The listing builds one solid part. Answer for the finished solid, in the listing's coordinates (mm). Face numbers are marked on the shaded views. A direction names the side the tool comes from. Give positions to 0.01 mm unless a question says otherwise; leave off trailing zeros. Loops run counter-clockwise (first coordinate to the right, second up) from the corner with the lowest first, then second, coordinate; pieces in that order, holes last. Notation, with made-up numbers: (71, -25.5) - (123, -25.5) arc R30 ccw to (123, 10.5) - close; hole circle Ø2 at (51.25, 29). An arc over 180 degrees is marked (long way). Write item = value, one per line. Start each with the question number.
1) The part is cut by section D-D on z = 0. Write down the section's boundary in (x, y), plus the area to 3 significant figures.
2) The part is cut by section A-A on y = -17.75. Write down the section's boundary in (x, z).
3) Flat-ended cylindrical pins translate along their axes: P1, Ø2.5, axis at x = -38.5, y = -12, coming from the -Z side; P2, Ø10, axis at y = -21, z = 11.5, coming from the -X side; P3, Ø10, axis at x = -38.5, z = 28, coming from the -Y side; P4, Ø2.5, axis at y = -5, z = -33.5, coming from the -X side. Find the tip coordinate at first contact, or state that the pin passes through.
4) The part is cut by section B-B on z = -15.5. Write down the section's boundary in (x, y), plus the area to 3 significant figures.
5) The part is cut by section C-C on x = -40.5. Write down the section's boundary in (y, z), plus the area to 3 significant figures.
6) Consider probe 1 along X at (y, z) = (-4.25, -3.5); probe 2 along Z at (x, y) = (-40.5, -4.75); probe 3 along X at (y, z) = (-2.75, 33). Determine where each line is inside the solid, lowest interval first.
7) Which of the six approach directions +Z, -Z, +X, -X, +Y, -Y give full straight-line access (tool end or side, diameter ignored) to the marked faces 5, 6 and 7?
8) The mould has two halves that part along X. Classify the marked faces 1, 2, 3 and 4: +X half, -X half, draft (parallel to the pull), parting line (faces both ways), or undercut.
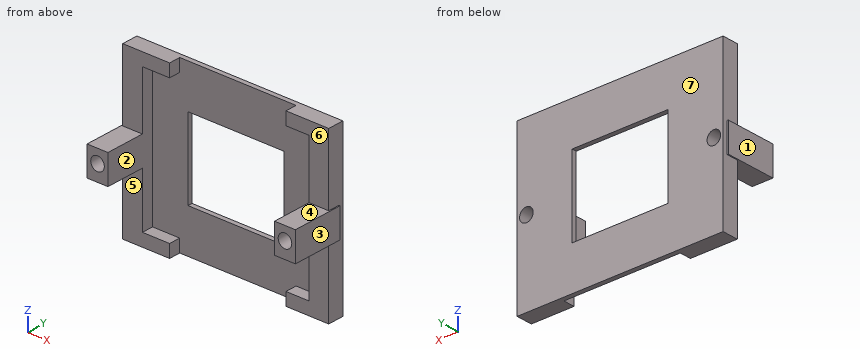
from build123d import *

# Parameters (mm, degrees)
F0_W      = 89
F0_H      = 72
F1_DEPTH  = 7
F2_W      = 72
F2_H      = 61
F3_DEPTH  = 5
F4_W      = 41.437034
F4_H      = 34.563594
F5_DEPTH  = 25
F6_W      = 50.274316
F6_H      = 5.5
F7_DEPTH  = 5
F8_W      = 9
F8_H      = 12.568578
F9_DEPTH  = 22
F10_R     = 2.9335
F11_DEPTH = 25


with BuildPart() as f1:
    # F0 (on Front) → F1 (new body)
    with BuildSketch(Plane.XZ):
        Rectangle(F0_W, F0_H)
    extrude(amount=F1_DEPTH)

    # F2 (on face) → F3 (cut)
    with BuildSketch(Plane.XZ.offset(7)):
        Rectangle(F2_W, F2_H)
    extrude(amount=-F3_DEPTH, mode=Mode.SUBTRACT)

    # F4 (on face) → F5 (cut)
    with BuildSketch(Plane.XZ.offset(2)):
        Rectangle(F4_W, F4_H)
    extrude(amount=-F5_DEPTH, mode=Mode.SUBTRACT)

    # F6 (on face) → F7 (cut)
    with BuildSketch(Plane.XZ.offset(7)):
        with Locations((0.883728, -33.25)):
            Rectangle(F6_W, F6_H)
        with Locations((0.883728, 33.25)):
            Rectangle(F6_W, F6_H)
    extrude(amount=-F7_DEPTH, mode=Mode.SUBTRACT)

    # F8 (on face) → F9 (join)
    with BuildSketch(Plane.XZ.offset(2)):
        with Locations((-40.5, -0.589152)):
            Rectangle(F8_W, F8_H)
        with Locations((40.5, -0.589152)):
            Rectangle(F8_W, F8_H)
    extrude(amount=F9_DEPTH)

    # F10 (on face) → F11 (cut)
    with BuildSketch(Plane.XZ.offset(24)):
        with Locations((-40.5, 0)):
            Circle(F10_R)
        with Locations((40.5, 0)):
            Circle(F10_R)
    extrude(amount=-F11_DEPTH, mode=Mode.SUBTRACT)


solid = f1.part
Answer below:
q1.outline = (-45, -24) - (-43.43, -24) - (-43.43, 0) - (-44.5, 0) - (-44.5, -2) - (-45, -2) - close; (-37.57, -24) - (-36, -24) - (-36, -2) - (-20.72, -2) - (-20.72, 0) - (-37.57, 0) - close; (20.72, -2) - (36, -2) - (36, -24) - (37.57, -24) - (37.57, 0) - (20.72, 0) - close; (43.43, -24) - (45, -24) - (45, -2) - (44.5, -2) - (44.5, 0) - (43.43, 0) - close
q1.area = 210 mm2
q2.outline = (-45, -6.87) - (-36, -6.87) - (-36, 5.7) - (-45, 5.7) - close; (36, -6.87) - (45, -6.87) - (45, 5.7) - (36, 5.7) - close; hole circle Ø5.87 at (-40.5, 0); hole circle Ø5.87 at (40.5, 0)
q3.P1 = -6.87
q3.P2 = through
q3.P3 = -7
q3.P4 = -44.5
q4.outline = (-44.5, -7) - (-36, -7) - (-36, -2) - (-20.72, -2) - (-20.72, 0) - (-44.5, 0) - close; (20.72, -2) - (36, -2) - (36, -7) - (44.5, -7) - (44.5, 0) - (20.72, 0) - close
q4.area = 180 mm2
q5.outline = (-24, -6.87) - (-7, -6.87) - (-7, -36) - (0, -36) - (0, -2.93) - (-24, -2.93) - close; (-24, 2.93) - (0, 2.93) - (0, 36) - (-7, 36) - (-7, 5.7) - (-24, 5.7) - close
q5.area = 577 mm2
q6.probe_1 = -45 to -36, 36 to 45
q6.probe_2 = -36 to -2.93, 2.93 to 36
q6.probe_3 = -44.5 to -24.25, 26.02 to 44.5
q7.face_5 = -Z, +X, -X, -Y
q7.face_6 = +Z, +X, -X, -Y
q7.face_7 = +Z, -Z, +X, -X, +Y
q8.face_1 = -X half
q8.face_2 = undercut
q8.face_3 = +X half
q8.face_4 = draft
